from build123d import *

# Parameters (mm, degrees)
P_IDAT_VYSUNUT_M1_DEPTH  = 70
ZAOBLIT1_R               = 35
ODEBRAT_VYSUNUT_M2_REACH = 166.125
SKICA3_R                 = 15
SKICA5_R                 = 20
ODEBRAT_VYSUNUT_M3_DEPTH = 5
ODEBRAT_VYSUNUT_M4_REACH = 166.125
SKICA6_R                 = 12.5
SKICA7_R                 = 18
ODEBRAT_VYSUNUT_M5_DEPTH = 9
SKICA8_R                 = 15
ODEBRAT_VYSUNUT_M6_DEPTH = 6
ODEBRAT_VYSUNUT_M7_REACH = 166.125
SKICA9_R                 = 18
SKICA10_R                = 21
ODEBRAT_VYSUNUT_M8_DEPTH = 5
ZKOSEN_1_SIZE            = 4


with BuildPart() as part:
    # Skica2 → Přidat vysunutím1 (new body)
    with BuildSketch(Plane.XY):
        Polygon((0, 0), (-121, 0), (-121, -86), (0, -86), (0, -68), (-100.200761753, -68), (-100.200761753, -18), (0, -18), align=None)
    extrude(amount=P_IDAT_VYSUNUT_M1_DEPTH)

    # Zaoblit1
    zaoblit1_edges = [part.edges().sort_by_distance(p)[0] for p in [
        (0, -77, 70),
        (0, -77, 0),
        (0, -9, 70),
        (0, -9, 0),
    ]]
    fillet(zaoblit1_edges, radius=ZAOBLIT1_R - 0.0001)  # a hair under: the kernel refuses the full size

    # Skica3 → Odebrat vysunutím2 (cut, up to next)
    with BuildSketch(Plane.ZY.offset(121), mode=Mode.PRIVATE) as odebrat_vysunut_m2_sk1:
        with Locations((35, -43)):
            Circle(SKICA3_R)
    odebrat_vysunut_m2_tool1 = extrude(odebrat_vysunut_m2_sk1.sketch, amount=-ODEBRAT_VYSUNUT_M2_REACH, mode=Mode.PRIVATE) & part.part
    add(odebrat_vysunut_m2_tool1.solids().sort_by_distance((-121, -43, 35))[0], mode=Mode.SUBTRACT)

    # Skica5 → Odebrat vysunutím3 (cut)
    with BuildSketch(Plane(origin=(-100.200761753, 0, 0), x_dir=(0, 0, -1), z_dir=(1, 0, 0))):
        with Locations((-35, -43)):
            Circle(SKICA5_R)
    extrude(amount=-ODEBRAT_VYSUNUT_M3_DEPTH, mode=Mode.SUBTRACT)

    # Skica6 → Odebrat vysunutím4 (cut, up to next)
    with BuildSketch(Plane(origin=(0, 0, 0), x_dir=(1, 0, 0), z_dir=(0, 1, 0)), mode=Mode.PRIVATE) as odebrat_vysunut_m4_sk1:
        with Locations(Location((-35, -35, 0), (0, 0, 180))):
            Circle(SKICA6_R)
    odebrat_vysunut_m4_tool1 = extrude(odebrat_vysunut_m4_sk1.sketch, amount=-ODEBRAT_VYSUNUT_M4_REACH, mode=Mode.PRIVATE) & part.part
    add(odebrat_vysunut_m4_tool1.solids().sort_by_distance((-35, 0, 35))[0], mode=Mode.SUBTRACT)

    # Skica7 → Odebrat vysunutím5 (cut)
    with BuildSketch(Plane(origin=(0, 0, 0), x_dir=(1, 0, 0), z_dir=(0, 1, 0))):
        with Locations(Location((-35, -35, 0), (0, 0, 180))):
            Circle(SKICA7_R)
    extrude(amount=-ODEBRAT_VYSUNUT_M5_DEPTH, mode=Mode.SUBTRACT)

    # Skica8 → Odebrat vysunutím6 (cut)
    with BuildSketch(Plane.XZ.offset(18)):
        with Locations(Location((-35, 35, 0), (0, 0, 270))):
            Circle(SKICA8_R)
    extrude(amount=-ODEBRAT_VYSUNUT_M6_DEPTH, mode=Mode.SUBTRACT)

    # Skica9 → Odebrat vysunutím7 (cut, up to next)
    with BuildSketch(Plane.XZ.offset(86), mode=Mode.PRIVATE) as odebrat_vysunut_m7_sk1:
        with Locations(Location((-35, 35, 0), (0, 0, 180))):
            Circle(SKICA9_R)
    odebrat_vysunut_m7_tool1 = extrude(odebrat_vysunut_m7_sk1.sketch, amount=-ODEBRAT_VYSUNUT_M7_REACH, mode=Mode.PRIVATE) & part.part
    add(odebrat_vysunut_m7_tool1.solids().sort_by_distance((-35, -86, 35))[0], mode=Mode.SUBTRACT)

    # Skica10 → Odebrat vysunutím8 (cut)
    with BuildSketch(Plane.XZ.offset(86)):
        with Locations((-35, 35)):
            Circle(SKICA10_R)
    extrude(amount=-ODEBRAT_VYSUNUT_M8_DEPTH, mode=Mode.SUBTRACT)

    # Zkosení1
    zkosen_1_edges = [part.edges().sort_by_distance(p)[0] for p in [
        (-121, -86, 35),
        (-121, 0, 35),
    ]]
    chamfer(zkosen_1_edges, length=ZKOSEN_1_SIZE)


solid = part.part
Geometry check sheet. Reference: the model listing, model coordinates, mm. A direction names the side the tool comes from. Coordinates: 2 decimals unless noted, no trailing zeros. Order: outer loops, then holes, each group sorted by start corner. A loop starts at its lowest first (then second) coordinate and runs counter-clockwise, first axis right, second up. Notation, with made-up numbers: (-5.5, 89.5) - (11.5, 89.5) arc R27 ccw to (11.5, 115.5) - close; hole circle Ø9 at (82, -31.75). An arc over 180 degrees is marked (long way). Answer in a Markdown table with one row per item. Add a question column.
1) Set-up check for faces 1 (the flat face through (-22.7, -9, 31.3)), 2 (the cylindrical face through (-102.666, -36.993, 15.924)), 3 (the flat face through (-22.7, -12, 38.4)): record each of +Z, -Z, +X, -X, +Y, -Y from which the full face is reachable in a straight line by a thin tool's end or side.
2) Cross-section at C-C, the plane y = -43. Record the cut outline in (x, z).
3) Material ranges on line 1 along X through (y, z) = (-14.55, 35); line 2 along Y through (x, z) = (-73.5, 31.5); line 3 along Z through (x, y) = (-35, -10), recorded low to high. Write a range as [from, to].
4) Cross-section at A-A, the plane x = -71. Record the cut outline in (y, z), then the cut area to 3 significant figures.
5) Cross-section at D-D, the plane z = 46. State how many separate pieces and enclosed holes the cut face has, then the cut area to 3 significant figures.
6) Release check for a two-part mould opening along Y. For faces 4 (the flat face through (-100.201, -21, 35)), 5 (the cylindrical face through (-52.169, -74.591, 29.593)), 6 (the flat face through (-105.201, -28, 32)), 7 (the flat face through (-71, 0, 35)) record: +Y half, -Y half, draft (parallel to the pull), parting line (faces both ways), or undercut.
7) Gauge pin test, flat ends, axial feed: P1, Ø12, axis at y = -49, z = 27.5, coming from the +X side; P2, Ø6, axis at y = -73, z = 40.5, coming from the +X side. Record the tip position at first contact, or that the pin passes through.
Check result:
| question | item | result |
|---|---|---|
| 1 | face 1 | +Y |
| 1 | face 2 | +X |
| 1 | face 3 | -Y |
| 2 | outline | (-121, 0) - (-100.2, 0) - (-100.2, 15) - (-105.2, 15) - (-105.2, 20) - (-121, 20) - close; (-121, 50) - (-105.2, 50) - (-105.2, 55) - (-100.2, 55) - (-100.2, 70) - (-121, 70) - close |
| 3 | line 1 | x = [-121, -50], [-20, 0] |
| 3 | line 2 | y = [-86, -68], [-18, 0] |
| 3 | line 3 | z = [0, 22.5], [47.5, 70] |
| 4 | outline | (-86, 0) - (-68, 0) - (-68, 70) - (-86, 70) - close; (-18, 0) - (0, 0) - (0, 70) - (-18, 70) - close |
| 4 | area | 2,520 mm² |
| 5 | separate pieces | 4 |
| 5 | enclosed holes | 0 |
| 5 | area | 3,860 mm² |
| 6 | face 4 | undercut |
| 6 | face 5 | draft |
| 6 | face 6 | undercut |
| 6 | face 7 | +Y half |
| 7 | P1 | stops at x = -105.2 |
| 7 | P2 | stops at x = -0.09 |
